Autodesk Fusion 360 part; units mm, degrees
sketch "草图1" plane through (0, 0, 0) normal (0, 0, 1) x (1, 0, 0)
  line L0 (7, 0) -> (124, 0)
  line L1 (131, 7) -> (131, 168)
  line L2 (0, 168) -> (0, 7)
  line L3 (14, 165) -> (117, 165)
  line L4 (12, 167) -> (12, 173)
  line L5 (119, 167) -> (119, 173)
  arc A0 (7, 175) -> (0, 168) centre (7, 168) ccw
  arc A1 (131, 168) -> (124, 175) centre (124, 168) ccw
  circle A2 centre (7, 168) radius 2
  circle A3 centre (7, 168) radius 2.5
  circle A4 centre (7, 168) radius 3.7
  circle A5 centre (124, 168) radius 2
  circle A6 centre (124, 168) radius 2.5
  circle A7 centre (124, 168) radius 3.7
  line L6 (7, 175) -> (10, 175)
  line L7 (121, 175) -> (124, 175)
  arc A8 (121, 175) -> (119, 173) centre (121, 173) ccw
  arc A9 (117, 165) -> (119, 167) centre (117, 167) ccw
  arc A10 (12, 173) -> (10, 175) centre (10, 173) ccw
  arc A11 (12, 167) -> (14, 165) centre (14, 167) ccw
  arc A12 (0, 7) -> (7, 0) centre (7, 7) ccw
  arc A13 (124, 0) -> (131, 7) centre (124, 7) ccw
  circle A14 centre (7, 7) radius 2
  circle A15 centre (7, 7) radius 2.5
  circle A16 centre (7, 7) radius 3.7
  circle A17 centre (124, 7) radius 2
  circle A18 centre (124, 7) radius 2.5
  circle A19 centre (124, 7) radius 3.7
  line L8 (11, 14.0612) -> (120, 14.0612)
  line L9 (124, 18.0612) -> (124, 71.0612)
  line L10 (120, 75.0612) -> (11, 75.0612)
  line L11 (7, 71.0612) -> (7, 18.0612)
  line L12 (12, 16) -> (119, 16)
  line L13 (122, 19) -> (122, 70)
  line L14 (119, 73) -> (12, 73)
  line L15 (9, 70) -> (9, 19)
  arc A20 (11, 75.0612) -> (7, 71.0612) centre (11, 71.0612) ccw
  arc A21 (12, 73) -> (9, 70) centre (12, 70) ccw
  arc A22 (124, 71.0612) -> (120, 75.0612) centre (120, 71.0612) ccw
  arc A23 (122, 70) -> (119, 73) centre (119, 70) ccw
  arc A24 (7, 18.0612) -> (11, 14.0612) centre (11, 18.0612) ccw
  arc A25 (9, 19) -> (12, 16) centre (12, 19) ccw
  arc A26 (120, 14.0612) -> (124, 18.0612) centre (120, 18.0612) ccw
  arc A27 (119, 16) -> (122, 19) centre (119, 19) ccw
  line L16 (9, 155) -> (122, 155)
  line L17 (124, 153) -> (124, 93)
  line L18 (122, 91) -> (9, 91)
  line L19 (7, 93) -> (7, 153)
  line L20 (10, 153) -> (121, 153)
  line L21 (122, 152) -> (122, 94)
  line L22 (121, 93) -> (10, 93)
  line L23 (9, 94) -> (9, 152)
  arc A28 (9, 155) -> (7, 153) centre (9, 153) ccw
  arc A29 (124, 153) -> (122, 155) centre (122, 153) ccw
  arc A30 (7, 93) -> (9, 91) centre (9, 93) ccw
  arc A31 (122, 91) -> (124, 93) centre (122, 93) ccw
  arc A32 (10, 153) -> (9, 152) centre (10, 152) ccw
  arc A33 (9, 94) -> (10, 93) centre (10, 94) ccw
  arc A34 (122, 152) -> (121, 153) centre (121, 152) ccw
  arc A35 (121, 93) -> (122, 94) centre (121, 94) ccw
  circle A36 centre (11, 151) radius 1.9
  line L24 (15, 151) -> (15, 153)
  line L25 (11, 147) -> (9, 147)
  circle A37 centre (11, 95) radius 1.9
  line L26 (11, 99) -> (9, 99)
  line L27 (15, 93) -> (15, 95)
  circle A38 centre (120, 95) radius 1.9
  line L28 (116, 95) -> (116, 93)
  line L29 (120, 99) -> (122, 99)
  circle A39 centre (120, 151) radius 1.9
  line L30 (116, 151) -> (116, 153)
  line L31 (120, 147) -> (122, 147)
  circle A40 centre (11, 71) radius 1.9
  line L32 (15, 71) -> (15, 73)
  line L33 (11, 67) -> (9, 67)
  arc A41 (11, 67) -> (15, 71) centre (11, 71) ccw
  circle A42 centre (11, 18) radius 1.9
  line L34 (11, 22) -> (9, 22)
  line L35 (15, 16) -> (15, 18)
  arc A43 (15, 18) -> (11, 22) centre (11, 18) ccw
  arc A44 (15, 95) -> (11, 99) centre (11, 95) ccw
  arc A45 (11, 147) -> (15, 151) centre (11, 151) ccw
  arc A46 (116, 151) -> (120, 147) centre (120, 151) ccw
  arc A47 (120, 99) -> (116, 95) centre (120, 95) ccw
  circle A48 centre (120, 18) radius 1.9
  line L36 (116, 18) -> (116, 16)
  line L37 (120, 22) -> (122, 22)
  arc A49 (120, 22) -> (116, 18) centre (120, 18) ccw
  circle A50 centre (120, 70.9999) radius 1.9
  line L38 (116, 71) -> (116, 73)
  line L39 (120, 67) -> (122, 67)
  arc A51 (116, 71) -> (120, 67) centre (120, 71) ccw
  point P0 (131, 0)
  point P1 (0, 175)
  point P2 (12, 165)
  point P3 (119, 165)
  point P4 (7, 14.0612)
  point P5 (124, 14.0612)
  point P6 (7, 75.0612)
  point P7 (9, 16)
  point P8 (122, 16)
  point P9 (9, 73)
  point P10 (7, 155)
  point P11 (124, 155)
  point P12 (7, 91)
  point P13 (9, 153)
  point P14 (122, 153)
  point P15 (9, 93)
  dimension "d1" = 131
  dimension "d2" = 175
  dimension "d3" = 107
  dimension "d4" = 7
  dimension "d5" = 7
  dimension "d6" = 4
  dimension "d7" = 5
  dimension "d8" = 7.4
  dimension "d9" = 4
  dimension "d10" = 5
  dimension "d11" = 7.4
  dimension "d12" = 2
  dimension "d13" = 2
  dimension "d14" = 2
  dimension "d15" = 2
  dimension "d16" = 7
  dimension "d17" = 7
  dimension "d18" = 4
  dimension "d19" = 5
  dimension "d20" = 7.4
  dimension "d21" = 4
  dimension "d22" = 5
  dimension "d23" = 7.4
  dimension "d24" = 117
  dimension "d25" = 61
  dimension "d26" = 113
  dimension "d27" = 57
  dimension "d28" = 4
  dimension "d29" = 3
  dimension "d30" = 4
  dimension "d31" = 3
  dimension "d32" = 4
  dimension "d33" = 3
  dimension "d34" = 4
  dimension "d35" = 3
  dimension "d36" = 117
  dimension "d37" = 64
  dimension "d38" = 113
  dimension "d39" = 60
  dimension "d40" = 2
  dimension "d41" = 2
  dimension "d42" = 2
  dimension "d43" = 2
  dimension "d44" = 1
  dimension "d45" = 1
  dimension "d46" = 1
  dimension "d47" = 1
  dimension "d57" = 3.8
  dimension "d58" = 3.8
  dimension "d59" = 3.8
  dimension "d60" = 3.8
  dimension "d62" = 3.8
  dimension "d63" = 4
  dimension "d64" = 3.8
  dimension "d65" = 4
  dimension "d66" = 4
  dimension "d68" = 4
  dimension "d69" = 4
  dimension "d70" = 3.8
  dimension "d71" = 4
  dimension "d72" = 3.8
  dimension "d73" = 4
extrude "拉伸13" cut sketch "草图1" along normal blind 16 contours A25 A42 picked at (9.8084, 16.8084)
extrude "拉伸14" cut sketch "草图1" along normal blind 16 contours A21 A40 picked at (10.7309, 71.3245)
extrude "拉伸15" cut sketch "草图1" along normal blind 16 contours A23 A50 picked at (121.1681, 72.2139)
extrude "拉伸16" cut sketch "草图1" along normal blind 16 contours A27 A48 picked at (120.3296, 17.7354)
extrude "拉伸17" add sketch "草图1" along normal blind 2 separate body contours L0 L1 L2 L3 L4 L5 A0 A1 L6 L7 A8 A9 A10 A11 A12 A13 | A3 | A4 | A6 | A7 | A15 | A16 | A18 | A19
extrude "拉伸18" add sketch "草图1" along normal blind 6 contours L16 L17 L18 L19 A28 A29 A30 A31 | L20 L23 A32 L24 L25 A45 | L20 L21 A34 L30 L31 A46 | L22 L23 A33 L26 L27 A44 | L21 L22 A35 L28 L29 A47
extrude "拉伸19" add sketch "草图1" along normal blind 16 contours L8 L9 L10 L11 A20 A22 A24 A26 | L12 L15 A25 A42 L34 L35 A43 | L12 L13 A27 A48 L36 L37 A49 | L14 L15 A21 A40 L32 L33 A41 | L13 L14 A23 A50 L38 L39 A51
extrude "拉伸20" cut sketch "草图1" against normal blind 0.4 from surface at 2 contours A3
extrude "拉伸21" cut sketch "草图1" against normal blind 0.4 from surface at 2 contours A6
extrude "拉伸22" cut sketch "草图1" against normal blind 0.4 from surface at 2 contours A18
extrude "拉伸23" cut sketch "草图1" against normal blind 0.4 from surface at 2 contours A15
Could you check a few things on this model? Use its own coordinates, in mm. A direction names the side the tool comes from. Give positions to 0.01 mm unless a question says otherwise; leave off trailing zeros. Order: outer loops, then holes, each group sorted by start corner. A loop starts at its lowest first (then second) coordinate and runs counter-clockwise, first axis right, second up.
1. We'd pull the mould along Y, two halves only. Please class faces 1 (the cylindrical face through (8.203, 15.202, 8.902)), 2 (the flat face through (7, 45, 9)), 3 (the cylindrical face through (125.34, 170.11, 1.8)): pulls with the +Y half, pulls with the -Y half, needs draft (parallel to the pull), parting line crosses it, or undercut.
2. I need wall thicknesses on L1, parallel to Y at x = 11, z = 9.5; L2, parallel to Y at x = 124, z = 1; L3, parallel to Y at x = 97.5, z = 9. Which ranges of each line are inside material? Lowest first, please.
3. Suppose I cut it at C-C (z = 8.25). List the corners of the cut face in (x, y) for me.
4. For faces 4 (the flat face through (66, 91, 4)), 5 (the flat face through (6, 9, 1.6)), 6 (the cylindrical face through (117.203, 68.141, 7.888)), which set-ups out of +Z, -Z, +X, -X, +Y, -Y let a thin tool reach every point of the face, with its end or its side?
5. Will these pins go through, and if not, where does the flat tip stop? P1, Ø4, axis at x = 124, y = 8, coming from the +Z side; P2, Ø4.5, axis at x = 124, y = 7, coming from the +Z side; P3, Ø2, axis at y = 170.5, z = 1, coming from the -X side; P4, Ø0.6, axis at y = 93.5, z = 2, coming from the -X side.
6. Suppose I cut it at B-B (y = 119). List the corners of the cut face in (x, z) for me.
7. Suppose I cut it at A-A (x = 33). List the corners of the cut face in (y, z) for me.
Solved:
1. face 1: pulls with the -Y half
1. face 2: needs draft
1. face 3: undercut
2. L1: y = 14.06 to 16.1, 19.9 to 22, 67 to 69.1, 72.9 to 75.06
2. L2: y = 0 to 5, 9 to 166, 170 to 175
2. L3: y = 14.06 to 16, 73 to 75.06
3. outline: (7, 18.06) arc R4 ccw to (11, 14.06) - (120, 14.06) arc R4 ccw to (124, 18.06) - (124, 71.06) arc R4 ccw to (120, 75.06) - (11, 75.06) arc R4 ccw to (7, 71.06) - close; hole (9, 22) - (11, 22) arc R4 cw to (15, 18) - (15, 16) - (116, 16) - (116, 18) arc R4 cw to (120, 22) - (122, 22) - (122, 67) - (120, 67) arc R4 cw to (116, 71) - (116, 73) - (15, 73) - (15, 71) arc R4 cw to (11, 67) - (9, 67) - close; hole circle Ø3.8 at (11, 18); hole circle Ø3.8 at (11, 71); hole circle Ø3.8 at (120, 18); hole circle Ø3.8 at (120, 71)
4. face 4: +Z, +X, -X
4. face 5: +Z
4. face 6: +Z, -Z
5. P1: stops at z = 2
5. P2: stops at z = 1.6
5. P3: stops at x = 0.16
5. P4: stops at x = 0
6. outline: (0, 0) - (9, 0) - (9, 6) - (7, 6) - (7, 2) - (0, 2) - close; (122, 0) - (131, 0) - (131, 2) - (124, 2) - (124, 6) - (122, 6) - close
7. outline: (0, 0) - (16, 0) - (16, 16) - (14.06, 16) - (14.06, 2) - (0, 2) - close; (73, 0) - (93, 0) - (93, 6) - (91, 6) - (91, 2) - (75.06, 2) - (75.06, 16) - (73, 16) - close; (153, 0) - (165, 0) - (165, 2) - (155, 2) - (155, 6) - (153, 6) - close
